Autodesk Inventor part; units mm, degrees
ref_plane "YZ Plane" through (0, 0, 0) normal (1, 0, 0) x (0, 1, 0)
ref_plane "XZ Plane" through (0, 0, 0) normal (0, 1, 0) x (-1, 0, 0)
ref_plane "XY Plane" through (0, 0, 0) normal (0, 0, 1) x (1, 0, 0)
sketch "Sketch1" plane through (0, 0, 0) normal (0, 1, 0) x (-1, 0, 0)
  line L0 (0, 0) -> (19, 0)
  line L1 (19, 0) -> (19, -50)
  line L2 (19, -50) -> (0, -50)
  line L3 (0, -50) -> (0, 0)
  dimension "d0" = 50
  dimension "d1" = 19
extrude "Extrusion1" add sketch "Sketch1" along normal blind 2
sketch "Sketch2" plane through (0, 2, 0) normal (0, 1, 0) x (1, 0, 0)
  line L0 (-19, 20) -> (-16.5, 20)
  line L1 (-16.5, 20) -> (-16.5, 30)
  line L2 (-16.5, 30) -> (-19, 30)
  line L3 (-19, 30) -> (-19, 20)
  line L4 (-19, 0) -> (0, 0)
  line L5 (-19, 50) -> (-19, 0)
  line L6 (-2.5, 20) -> (0, 20)
  line L7 (0, 20) -> (0, 30)
  line L8 (0, 30) -> (-2.5, 30)
  line L9 (-2.5, 30) -> (-2.5, 20)
  line L10 (0, 0) -> (0, 50)
  dimension "d4" = 2.5
  dimension "d5" = 10
  dimension "d6" = 20
  dimension "d7" = 10
  dimension "d8" = 2.5
  dimension "d9" = 20
extrude "Extrusion2" cut sketch "Sketch2" against normal through all
sketch "Sketch3" plane through (-16.5, 2, -20) normal (0, 0, -1) x (-1, 0, 0)
  line L0 (2.5, 0) -> (-16.5, 0)
  arc A0 (0, 0) -> (-14, 0) centre (-7, 0) ccw
  point P0 (-16.5, -2)
  dimension "d12" = 7
extrude "Extrusion3" add sketch "Sketch3" along normal blind 10
sketch "Sketch5" plane through (0, 2, 0) normal (0, 1, 0) x (1, 0, 0)
  line L0 (-16.5, 20) -> (-19, 20)
  line L1 (-19, 20) -> (0, 20)
  line L2 (0, 20) -> (0, 18)
  line L3 (0, 18) -> (-19, 18)
  line L4 (-19, 18) -> (-19, 20)
  line L5 (-19, 30) -> (-16.5, 30)
  line L6 (-19, 30) -> (0, 30)
  line L7 (0, 30) -> (0, 32)
  line L8 (0, 32) -> (-19, 32)
  line L9 (-19, 32) -> (-19, 30)
  line L10 (0, 0) -> (0, 20)
  line L11 (0, 30) -> (0, 50)
  dimension "d15" = 2
  dimension "d16" = 2
extrude "Extrusion4" add sketch "Sketch5" along normal blind 2
sketch "Sketch6" plane through (-16.5, 2, -30) normal (0, 0, -1) x (-1, 0, 0)
  arc A0 (2, 2) -> (-16, 2) centre (-7, 2) ccw
  line L0 (2.5, 0) -> (2.5, 2)
  line L1 (-13.7082, 2) -> (-0.2918, 2)
  line L2 (2, 2) -> (-16, 2)
  point P0 (-16.5, -2)
  dimension "d19" = 9
  dimension "d21" = 0
  dimension "d22" = 0
  dimension "d23" = 9.5
  dimension "d24" = 0
extrude "Extrusion5" add sketch "Sketch6" along normal blind 2
sketch "Sketch7" plane through (-16.5, 2, -20) normal (0, 0, 1) x (1, 0, 0)
  arc A0 (16, 2) -> (-2, 2) centre (7, 2) ccw
  line L0 (-2.5, 2) -> (16.5, 2)
  point P0 (16.5, -2)
  point P1 (7, 2)
  point P2 (-2, 2)
  point P3 (16, 2)
  dimension "d27" = 9
  dimension "d28" = 0
  dimension "d29" = 0
extrude "Extrusion6" add sketch "Sketch7" along normal blind 2
sketch "Sketch8" plane through (0, 4, 0) normal (0, 1, 0) x (1, 0, 0)
  line L0 (0, 18) -> (-19, 18)
  line L1 (-19, 20) -> (-16.5, 20)
  line L2 (-19, 18) -> (-19, 20)
  line L3 (-19, 20) -> (-18.5, 20)
  line L4 (-18.5, 20) -> (-19, 18)
  line L5 (-0.5, 30) -> (-18.5, 30)
  line L6 (-19, 50) -> (-19, 32)
  line L7 (-18.5, 30) -> (-19, 32)
  line L8 (-19, 32) -> (-19, 30)
  line L9 (-19, 30) -> (-18.5, 30)
  line L10 (0, 20) -> (-0.5, 20)
  line L11 (-0.5, 20) -> (0, 20)
  line L12 (0, 18) -> (0, 20)
  line L13 (0, 20) -> (0, 18)
  line L14 (0, 18) -> (-0.5, 20)
  line L15 (0, 30) -> (-2.5, 30)
  line L16 (0, 30) -> (0, 32)
  line L17 (0, 32) -> (0, 30)
  line L18 (0, 30) -> (-0.5, 30)
  line L19 (-0.5, 32) -> (-0.5, 30)
  line L20 (-0.5, 30) -> (0, 32)
  point P0 (0, 0)
extrude "Extrusion7" cut sketch "Sketch8" against normal through all
sketch "Sketch9" plane through (0, 2, 0) normal (0, 1, 0) x (1, 0, 0)
  circle A0 centre (-9.5, 9) radius 2.25
  circle A1 centre (-9.5, 41) radius 2.25
  line L0 (-19, 0) -> (0, 0)
  line L1 (0, 50) -> (-19, 50)
  line L2 (-19, 18) -> (-19, 0)
  line L3 (-19, 50) -> (-19, 32)
  dimension "d34" = 4.5
  dimension "d35" = 4.5
  dimension "d36" = 9
  dimension "d37" = 9
  dimension "d38" = 9.5
  dimension "d39" = 9.5
extrude "Extrusion8" cut sketch "Sketch9" against normal through all
chamfer "Chamfer1" distance 1 angle 45 2 edges at (-11.75, 2, -9) (-11.75, 2, -41)
properties part number "SUPPORT_POULIE_ARRIERE"
CAD build for the part. Positions are in the model's coordinates, mm. A direction names the side the tool comes from. Give positions to 0.01 mm unless a question says otherwise; leave off trailing zeros. Write each loop counter-clockwise with the first axis right and the second up, starting at its lowest first coordinate (ties: lowest second). Pieces come first, ordered by that corner, then holes. Notation, with made-up numbers: M 5.5,-7.5 L 63.5,-7.5 A20 ccw 63.5,0.5 Z; hole C 4,9 d1. An arc over 180 degrees is marked long. Return JSON: item names as keys, results as strings. Group by question number.
(1) Drill centre lines: L1, parallel to Z at x = -9.5, y = 0.6; L2, parallel to X at y = 0.2, z = -9; L3, parallel to Z at x = -4, y = 11. Where is each one in solid material? Low to high. Write a range as [from, to].
(2) Band-saw the part on D-D (x = -2). Give the cut face in (y, z).
(3) Flat gauge pins, fed straight in: pin 1 Ø6 at (y, z) = (11.5, -29) entering from +X; pin 2 Ø5.5 at (x, z) = (-7.5, -9.5) entering from +Y; pin 3 Ø1 at (x, y) = (-9.5, 7) entering from +Z. Where does each tip first touch, or does it go through?
(4) Mould opens along Z. For faces 6 (the face through (-9, 2, -13)), 7 (the face through (-9, 6, -32)), 8 (the face through (-2.5, 1, -25)) say: pulls with the +Z half, pulls with the -Z half, needs draft (parallel to the pull), parting line crosses it, or undercut.
(5) Band-saw the part on A-A (z = -9). Give the cut face in (x, y).
(6) Band-saw the part on B-B (x = -9.5). Give the cut face in (y, z), and give its area (3 significant figures).
(7) 3-axis set-ups, long thin cutter, end or side, ignore diameter. For faces 1 (the face through (-9.35, 9, -24.93)), 2 (the face through (-9, 2, -37)), 3 (the face through (0, 1, -41)), 4 (the face through (-18.746, 2.028, -19.014)), 5 (the face through (-0.253, 2.028, -30.986)): which of +Z, -Z, +X, -X, +Y, -Y reach the whole face in a straight line?
(8) Band-saw the part on C-C (y = 11). Give the cut face in (x, z), and give its area (3 significant figures).
Entries:
{
 "1": {"L1": "z = [-50, -43.25], [-38.75, -11.25], [-6.75, 0]", "L2": "x = [-19, -11.75], [-7.25, 0]", "L3": "z = [-32, -30], [-20, -18]"},
 "2": {"outline": "M 0,-50 L 2,-50 L 2,-32 L 8.97,-32 L 8.97,-30 L 0,-30 Z; M 0,-20 L 8.97,-20 L 8.97,-18 L 2,-18 L 2,0 L 0,0 Z"},
 "3": {"pin 1": "stops at x = -1.81", "pin 2": "stops at y = 2", "pin 3": "stops at z = -18"},
 "4": {"face 6": "needs draft", "face 7": "pulls with the -Z half", "face 8": "undercut"},
 "5": {"outline": "M -19,0 L -11.75,0 L -11.75,1 L -12.75,2 L -19,2 Z; M -7.25,0 L 0,0 L 0,2 L -6.25,2 L -7.25,1 Z"},
 "6": {"outline": "M 0,-50 L 2,-50 L 2,-44.25 L 1,-43.25 L 0,-43.25 Z; M 0,-38.75 L 1,-38.75 L 2,-37.75 L 2,-32 L 13,-32 L 13,-30 L 9,-30 L 9,-20 L 13,-20 L 13,-18 L 2,-18 L 2,-12.25 L 1,-11.25 L 0,-11.25 Z; M 0,-6.75 L 1,-6.75 L 2,-5.75 L 2,0 L 0,0 Z", "area": "194 mm^2"},
 "7": {"face 1": "+Y", "face 2": "-Z, +X, -X, +Y", "face 3": "+Z, -Z, +X, +Y, -Y", "face 4": "-X, +Y, -Y", "face 5": "+X, +Y, -Y"},
 "8": {"outline": "M -15.16,-32 L -3.84,-32 L -3.84,-30 L -15.16,-30 Z; M -15.16,-20 L -3.84,-20 L -3.84,-18 L -15.16,-18 Z", "area": "45.3 mm^2"}
}
